Answer from the drawing. Dimensions are ordinates in mm from the lowest x, y and z of the part. Coordinates: 2 decimals unless noted, no trailing zeros. Order: outer loops, then holes, each group sorted by start corner. A loop starts at its lowest first (then second) coordinate and runs counter-clockwise, first axis right, second up. Notation, with made-up numbers: (51, -6) - (77, -6) arc R14 cw to (77, 5) - close; hole circle Ø8 at (52.25, -3.5). An arc over 180 degrees is marked (long way). Use a Markdown table: item, result. Add a question column.
Item 1: Find the intervals of material crossed by line 1 along Z through (x, y) = (29, 2.7) (1 decimal); line 2 along X through (y, z) = (2.85, 22.5) (1 decimal); line 3 along Z through (x, y) = (30, 1.75) (1 decimal), in increasing order.
Item 2: A flat-ended cylindrical pin translates along its axis: P1, Ø12, axis at x = 14.5, z = 12.5, coming from the +Y side. Find the tip coordinate at first contact, or state that the pin passes through.
Item 3: The part is cut by section A-A, the plane x = 17.5. Give the vertices of the cut face in (y, z).
Item 4: The part is cut by section D-D, the plane x = 26. Give the vertices of the cut face in (y, z) (1 decimal).
Item 5: The mould has two halves that part along X. Classify the marked faces 1, 2 and 3: released by +X, released by -X, zero draft, split by the parting line, or undercut.
Item 6: The part is cut by section B-B, the plane y = 2. Give the vertices of the cut face in (x, z) (1 decimal).
Item 7: The part is cut by section C-C, the plane z = 27.5. Give the vertices of the cut face in (x, y) (1 decimal).
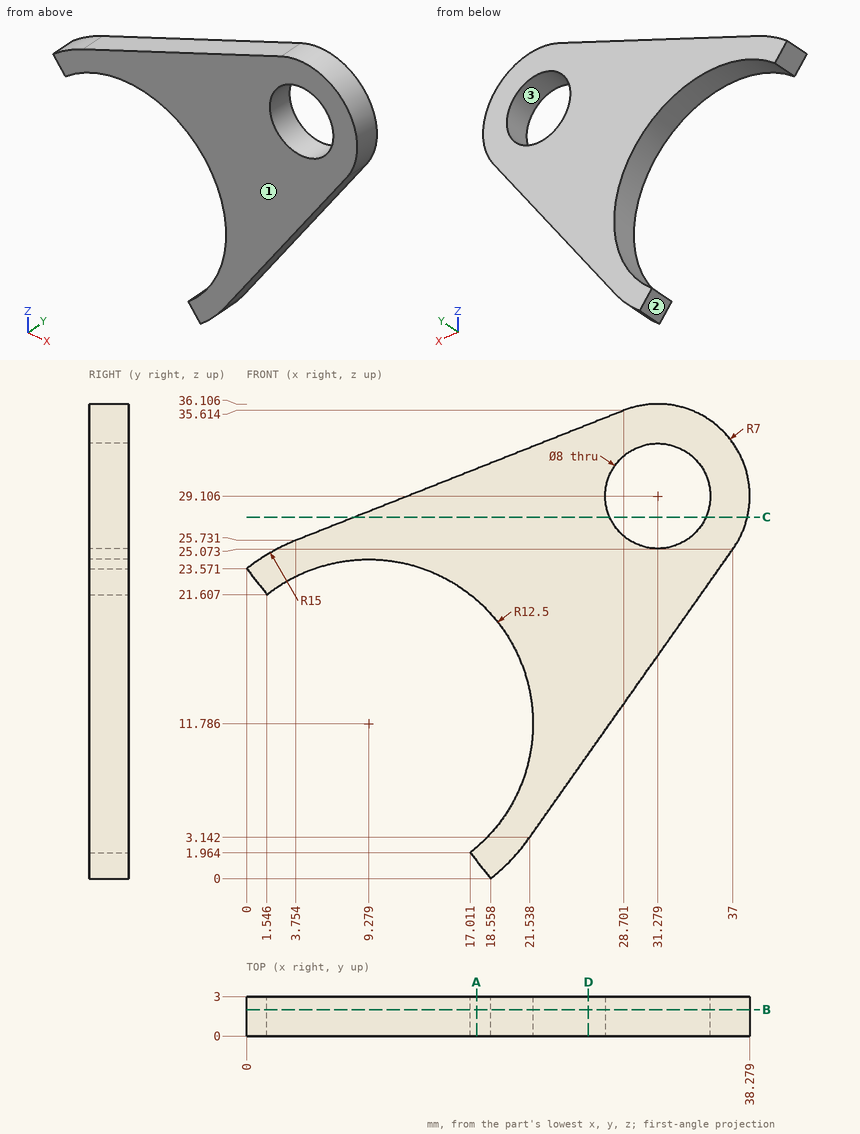
Solution:
| question | item | result |
|---|---|---|
| 1 | line 1 | z = 13.7 to 25.8, 32.4 to 35.7 |
| 1 | line 2 | x = 0.8 to 2.8, 15.7 to 35.2 |
| 1 | line 3 | z = 15.1 to 25.3, 32.9 to 36 |
| 2 | P1 | passes through |
| 3 | outline | (0, 1.34) - (3, 1.34) - (3, 2.37) - (0, 2.37) - close; (0, 21.2) - (3, 21.2) - (3, 31.18) - (0, 31.18) - close |
| 4 | outline | (0, 9.5) - (3, 9.5) - (3, 34.5) - (0, 34.5) - close |
| 5 | face 1 | zero draft |
| 5 | face 2 | released by -X |
| 5 | face 3 | undercut |
| 6 | outline | (0, 23.6) - (1.5, 21.6) arc R12.5 cw to (17, 2) - (18.6, 0) arc R15 ccw to (21.5, 3.1) - (37, 25.1) arc R7 ccw to (28.7, 35.6) - (3.8, 25.7) arc R15 ccw to start; hole circle Ø8 at (31.3, 29.1) |
| 7 | outline | (8.2, 0) - (27.6, 0) - (27.6, 3) - (8.2, 3) - close; (34.9, 0) - (38.1, 0) - (38.1, 3) - (34.9, 3) - close |
